from build123d import *

# Parameters (mm, degrees)
SKETCH1_R           = 1.6
SKETCH1_R_2         = 2.1
SKETCH1_R_3         = 4
BOSS_EXTRUDE1_DEPTH = 4


with BuildPart() as part:
    # Sketch1 → Boss-Extrude1 (new body)
    with BuildSketch(Plane(origin=(0, 0, 0), x_dir=(1, 0, 0), z_dir=(0, 1, 0))):
        with BuildLine():
            Line((-35, -26), (35, -26))
            ThreePointArc((35, -26), (38.535533906, -24.535533906), (40, -21))
            Line((40, -21), (40, 0))
            ThreePointArc((40, 0), (38.535533906, 3.535533906), (35, 5))
            Line((35, 5), (12.5, 5))
            Line((12.5, 5), (12.5, 20))
            Line((12.5, 20), (-12.5, 20))
            Line((-12.5, 20), (-12.5, 5))
            Line((-12.5, 5), (-35, 5))
            ThreePointArc((-35, 5), (-38.535533906, 3.535533906), (-40, 0))
            Line((-40, 0), (-40, -21))
            ThreePointArc((-40, -21), (-38.535533906, -24.535533906), (-35, -26))
        make_face()
        with Locations((-7.5, 11)):
            Circle(SKETCH1_R, mode=Mode.SUBTRACT)
        with Locations((7.5, 11)):
            Circle(SKETCH1_R, mode=Mode.SUBTRACT)
        with Locations((-7.5, -5)):
            Circle(SKETCH1_R, mode=Mode.SUBTRACT)
        with Locations((7.5, -5)):
            Circle(SKETCH1_R, mode=Mode.SUBTRACT)
        with Locations((-7.5, 5)):
            Circle(SKETCH1_R, mode=Mode.SUBTRACT)
        with Locations((7.5, 5)):
            Circle(SKETCH1_R, mode=Mode.SUBTRACT)
        with Locations((-35, -20)):
            Circle(SKETCH1_R, mode=Mode.SUBTRACT)
        with Locations((35, -20)):
            Circle(SKETCH1_R, mode=Mode.SUBTRACT)
        with Locations((-25, -10)):
            Circle(SKETCH1_R_2, mode=Mode.SUBTRACT)
        with Locations((25, -10)):
            Circle(SKETCH1_R_2, mode=Mode.SUBTRACT)
        with Locations((0, -20)):
            Circle(SKETCH1_R_3, mode=Mode.SUBTRACT)
    extrude(amount=BOSS_EXTRUDE1_DEPTH)


solid = part.part
Source: CAD feature listing. Evaluate the final solid. Frame: model axes, mm. A direction names the side the tool comes from. Coordinates: 2 decimals unless noted, no trailing zeros. Loops run counter-clockwise (first coordinate to the right, second up) from the corner with the lowest first, then second, coordinate; pieces in that order, holes last. Notation, with made-up numbers: (48.25, -9.75) -> (91.25, -9.75) arc R15 ccw to (91.25, -1.75) -> close; hole circle Ø1 at (-19.5, 25). An arc over 180 degrees is marked (long way). Answer in a Markdown table with one row per item. Add a question column.
Q1. Pull-direction query (X, two-part tool) for faces 4 (the face through (-12.5, 2, -13)), 5 (the face through (-9.1, 1.97, -11.07)), 6 (the face through (0, 2, -20)), 7 (the face through (-35.208, 1.972, 18.414)); classes: pulls with the +X half, pulls with the -X half, needs draft (parallel to the pull), parting line crosses it, or undercut.
Q2. Section C-C on z = -11. Return the cut outline in (x, y).
Q3. Reachability of faces 1 (the face through (5.9, 1.97, -11.07)), 2 (the face through (12.5, 2, -12)), 3 (the face through (-24, 2, -5)) from +Z, -Z, +X, -X, +Y, -Y: full face, straight path, thin tool, end or side. Return the list, or none.
Q4. Section B-B on y = 2.6. Give the number of separate pieces and of enclosed holes in the cut face, and give its area (3 significant figures).
Q5. Section A-A on x = -7.5. Return the cut outline in (y, z).
Q6. Contact query for flat-ended pins moving along their axis: pin 1 Ø3 at (x, z) = (-7.5, 5) entering from +Y; pin 2 Ø10 at (x, z) = (-13, -11) entering from +Y; pin 3 Ø2 at (y, z) = (3, -12) entering from +X; pin 4 Ø2 at (x, y) = (-27.5, 1.5) entering from -Z. Output: stop coordinate, or through.
Q7. Section D-D on x = 25. Return the cut outline in (y, z), and give its area (3 significant figures).
Q8. Ray query, line 1 along Z through (x, y) = (7.5, 1.8); line 2 along X through (y, z) = (0.8, 10); line 3 along X through (y, z) = (1.4, 5). Return the intervals inside material, ascending.
Computed values:
| question | item | result |
|---|---|---|
| 1 | face 4 | pulls with the -X half |
| 1 | face 5 | undercut |
| 1 | face 6 | needs draft |
| 1 | face 7 | undercut |
| 2 | outline | (-12.5, 0) -> (-9.1, 0) -> (-9.1, 4) -> (-12.5, 4) -> close; (-5.9, 0) -> (5.9, 0) -> (5.9, 4) -> (-5.9, 4) -> close; (9.1, 0) -> (12.5, 0) -> (12.5, 4) -> (9.1, 4) -> close |
| 3 | face 1 | +Y, -Y |
| 3 | face 2 | -Z, +X, +Y, -Y |
| 3 | face 3 | -Z, -X, +Y, -Y |
| 4 | separate pieces | 1 |
| 4 | enclosed holes | 11 |
| 4 | area | 2,690 mm^2 |
| 5 | outline | (0, -20) -> (4, -20) -> (4, -12.6) -> (0, -12.6) -> close; (0, -9.4) -> (4, -9.4) -> (4, -6.6) -> (0, -6.6) -> close; (0, -3.4) -> (4, -3.4) -> (4, 3.4) -> (0, 3.4) -> close; (0, 6.6) -> (4, 6.6) -> (4, 26) -> (0, 26) -> close |
| 6 | pin 1 | passes through |
| 6 | pin 2 | stops at y = 4 |
| 6 | pin 3 | stops at x = 12.5 |
| 6 | pin 4 | stops at z = -5 |
| 7 | outline | (0, -5) -> (4, -5) -> (4, 7.9) -> (0, 7.9) -> close; (0, 12.1) -> (4, 12.1) -> (4, 26) -> (0, 26) -> close |
| 7 | area | 107 mm^2 |
| 8 | line 1 | z = -20 to -12.6, -9.4 to -6.6, -3.4 to 3.4, 6.6 to 26 |
| 8 | line 2 | x = -40 to -27.1, -22.9 to 22.9, 27.1 to 40 |
| 8 | line 3 | x = -40 to -9.1, -5.9 to 5.9, 9.1 to 40 |
